from build123d import *

# Parameters (mm, degrees)
SKETCH1_W           = 19.05
SKETCH1_H           = 19.05
BOSS_EXTRUDE1_DEPTH = 19.05
SKETCH2_W           = 15.875
SKETCH2_H           = 15.875
BOSS_EXTRUDE2_DEPTH = 28.575
SKETCH3_W           = 15.875
SKETCH3_H           = 15.875
BOSS_EXTRUDE3_DEPTH = 28.575
SKETCH4_W           = 15.875
SKETCH4_H           = 15.875
BOSS_EXTRUDE4_DEPTH = 28.575
SKETCH5_W           = 15.875
SKETCH5_H           = 15.875
BOSS_EXTRUDE5_DEPTH = 28.575


with BuildPart() as part:
    # Sketch1 → Boss-Extrude1 (new body)
    with BuildSketch(Plane.XY):
        Rectangle(SKETCH1_W, SKETCH1_H)
    extrude(amount=BOSS_EXTRUDE1_DEPTH)

    # Sketch2 → Boss-Extrude2 (add)
    with BuildSketch(Plane(origin=(0, 9.525, 0), x_dir=(1, 0, 0), z_dir=(0, 1, 0))):
        with Locations((0, -9.525)):
            Rectangle(SKETCH2_W, SKETCH2_H)
    extrude(amount=BOSS_EXTRUDE2_DEPTH)

    # Sketch3 → Boss-Extrude3 (add)
    with BuildSketch(Plane(origin=(9.525, 0, 0), x_dir=(0, 0, -1), z_dir=(1, 0, 0))):
        with Locations((-9.525, 0)):
            Rectangle(SKETCH3_W, SKETCH3_H)
    extrude(amount=BOSS_EXTRUDE3_DEPTH)

    # Sketch4 → Boss-Extrude4 (add)
    with BuildSketch(Plane.XY.offset(19.05)):
        Rectangle(SKETCH4_W, SKETCH4_H)
    extrude(amount=BOSS_EXTRUDE4_DEPTH)

    # Sketch5 → Boss-Extrude5 (add)
    with BuildSketch(Plane.ZY.offset(9.525)):
        with Locations((9.525, 0)):
            Rectangle(SKETCH5_W, SKETCH5_H)
    extrude(amount=BOSS_EXTRUDE5_DEPTH)


solid = part.part
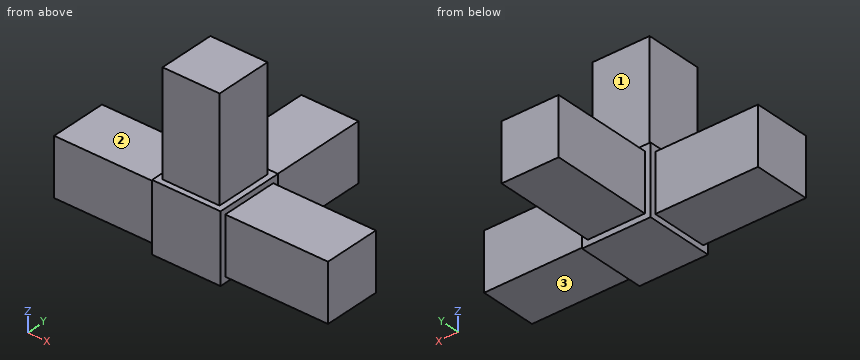
Geometry: final body of the model. Coordinates: model frame, mm. Face numbers are marked on the shaded views. A direction names the side the tool comes from. Give positions to 0.01 mm unless a question says otherwise; leave off trailing zeros. Loops run counter-clockwise (first coordinate to the right, second up) from the corner with the lowest first, then second, coordinate; pieces in that order, holes last. Notation, with made-up numbers: (62.25, 42) - (71.25, 42) arc R18 cw to (71.25, 46) - close; hole circle Ø6 at (53.5, 84.25). An arc over 180 degrees is marked (long way). One line per question, with ' | ' between items. Start each with the question number.
(1) Reachability of the marked faces 1, 2 and 3 from +Z, -Z, +X, -X, +Y, -Y: full face, straight path, thin tool, end or side. Return the list, or none.
(2) Contact query for flat-ended pins moving along their axis: pin 1 (17.5 mm diameter, centred on x = -18, y = 3, fed in from -Z); pin 2 (1 mm diameter, centred on x = -9.5, y = 20, fed in from -Z); pin 3 (5 mm diameter, centred on x = 28, y = -0.5, fed in from -Z); pin 4 (12.5 mm diameter, centred on x = -25.5, z = 13, fed in from -Y). Output: stop coordinate, or through.
(3) Section query A-A on z = 7. Return loops of the section in (x, y) (1 decimal).
(4) Section query D-D on x = 12. Return loops of the section in (y, z), then the cut area to 3 significant figures.
(5) Ray query, line 1 (Y direction, x = -14, z = 11.5); line 2 (Z direction, x = 16.5, y = -2). Return the intervals inside material, ascending. Write a range as from..to.
The answers:
1) face 1: +Z, +X, -X, +Y | face 2: +Z, -X, +Y, -Y | face 3: -Z, +X, +Y, -Y
2) pin 1: z = 0 | pin 2: through | pin 3: z = 1.59 | pin 4: y = -7.94
3) outline: (-38.1, -7.9) - (-9.5, -7.9) - (-9.5, -9.5) - (9.5, -9.5) - (9.5, -7.9) - (38.1, -7.9) - (38.1, 7.9) - (9.5, 7.9) - (9.5, 9.5) - (7.9, 9.5) - (7.9, 38.1) - (-7.9, 38.1) - (-7.9, 9.5) - (-9.5, 9.5) - (-9.5, 7.9) - (-38.1, 7.9) - close
4) outline: (-7.94, 1.59) - (7.94, 1.59) - (7.94, 17.46) - (-7.94, 17.46) - close | area: 252 mm2
5) line 1: -7.94..7.94 | line 2: 1.59..17.46
